For this review, use the dimensioned drawing (mm, ordinates from the lowest corner) and the shaded views. A direction names the side the tool comes from. Give positions to 0.01 mm unless a question says otherwise; leave off trailing zeros. Loops run counter-clockwise (first coordinate to the right, second up) from the corner with the lowest first, then second, coordinate; pieces in that order, holes last. Notation, with made-up numbers: (54, 78.25) -> (105, 78.25) arc R11 cw to (105, 93.25) -> close; hole circle Ø1 at (69, -23). An arc over 180 degrees is marked (long way). Use a Markdown table: item, result. Add a question column.
1. Add section B-B (y = 14.5). State the section outline as (x, z) points, and give its area (3 significant figures).
2. For the marked faces 1, 2, 3 and 4, list the 3-axis set-ups (+Z, -Z, +X, -X, +Y, -Y) from which the entire face can be reached by the end or side of a thin tool; tool diameter is ignored.
3. For pin 1 Ø1.5 at (y, z) = (13, 11) entering from +X; pin 2 Ø1 at (x, z) = (16, 9) entering from -Y; pin 3 Ø2.5 at (x, y) = (2.05, 14.5) entering from +Z; pin 4 Ø1.7 at (x, y) = (2.05, 2.5) entering from +Z (1 decimal), all flat-tipped, find the tip position at first contact; note any pin that passes through.
4. Add section C-C (y = 2.5). State the section outline as (x, z) points.
5. To check wall thickness, follow line 1 (Y direction, x = 2.05, z = 1.7); line 2 (Z direction, x = 19, y = 4.75); line 3 (X direction, y = 14.5, z = 9). State the ranges of each line that lie inside material, in increasing order.
6. Add section D-D (x = 6.5). State the section outline as (y, z) points.
7. Add section A-A (x = 2.05). State the section outline as (y, z) points.
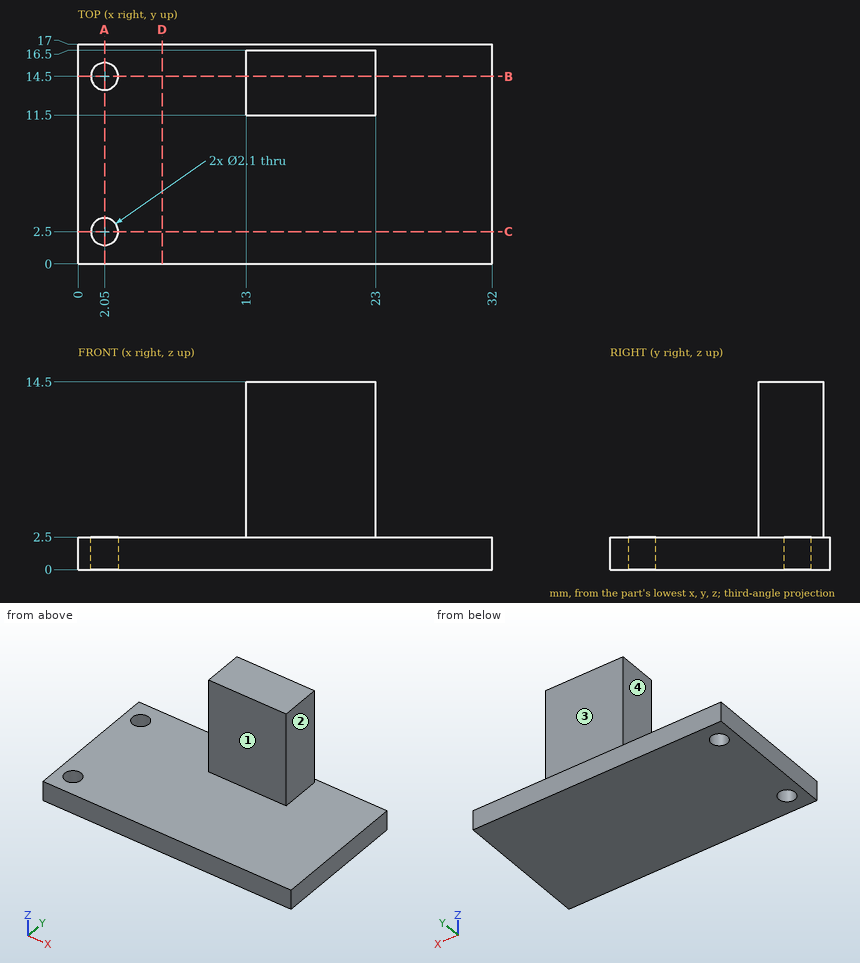
Taken from the geometry:
| question | item | result |
|---|---|---|
| 1 | outline | (0, 0) -> (1, 0) -> (1, 2.5) -> (0, 2.5) -> close; (3.1, 0) -> (32, 0) -> (32, 2.5) -> (23, 2.5) -> (23, 14.5) -> (13, 14.5) -> (13, 2.5) -> (3.1, 2.5) -> close |
| 1 | area | 195 mm^2 |
| 2 | face 1 | +Z, +X, -X, -Y |
| 2 | face 2 | +Z, +X, +Y, -Y |
| 2 | face 3 | +Z, +X, -X, +Y |
| 2 | face 4 | +Z, -X, +Y, -Y |
| 3 | pin 1 | stops at x = 23 |
| 3 | pin 2 | stops at y = 11.5 |
| 3 | pin 3 | stops at z = 2.5 |
| 3 | pin 4 | passes through |
| 4 | outline | (0, 0) -> (1, 0) -> (1, 2.5) -> (0, 2.5) -> close; (3.1, 0) -> (32, 0) -> (32, 2.5) -> (3.1, 2.5) -> close |
| 5 | line 1 | y = 0 to 1.45, 3.55 to 13.45, 15.55 to 17 |
| 5 | line 2 | z = 0 to 2.5 |
| 5 | line 3 | x = 13 to 23 |
| 6 | outline | (0, 0) -> (17, 0) -> (17, 2.5) -> (0, 2.5) -> close |
| 7 | outline | (0, 0) -> (1.45, 0) -> (1.45, 2.5) -> (0, 2.5) -> close; (3.55, 0) -> (13.45, 0) -> (13.45, 2.5) -> (3.55, 2.5) -> close; (15.55, 0) -> (17, 0) -> (17, 2.5) -> (15.55, 2.5) -> close |
